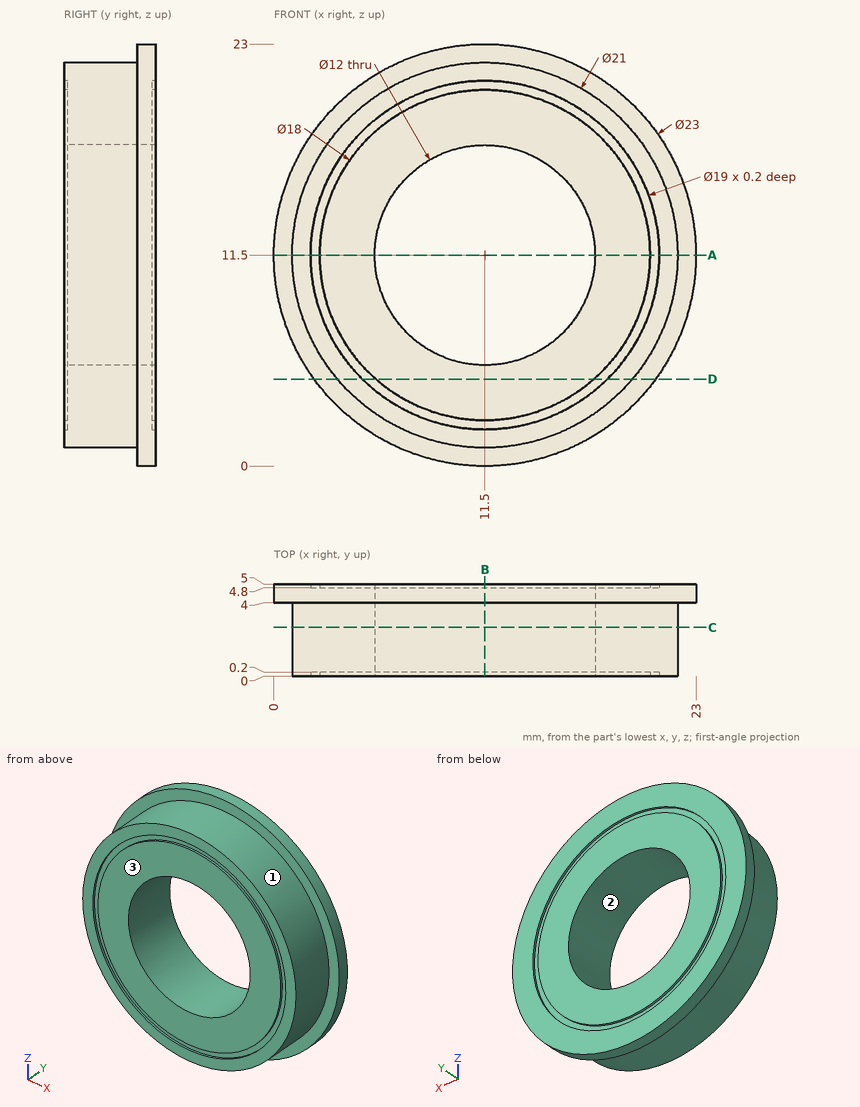
Drawing for the job (mm, zero at the part's lowest x, y, z). Coordinates: 2 decimals unless noted, no trailing zeros. Write each loop counter-clockwise with the first axis right and the second up, starting at its lowest first coordinate (ties: lowest second). Pieces come first, ordered by that corner, then holes. Notation, with made-up numbers: (-8.75, 2.25) -> (11.25, 2.25) arc R23 cw to (11.25, 19.25) -> close; hole circle Ø11 at (54.25, 30.25). An arc over 180 degrees is marked (long way). One line per item, written item: value. Start each with the question number.
1) Slice it at C-C on y = 2.65. Write the cut outline in (x, z).
2) Pull direction X, two halves, no side cores. Call the marked faces 1, 2 and 3: +X half, -X half, draft (parallel to the pull), parting line (faces both ways), or undercut.
3) Flat gauge pins, fed straight in: pin 1 Ø1 at (x, y) = (15.5, 1.5) entering from -Z; pin 2 Ø1.5 at (x, y) = (5, 1) entering from +Z. Where does each tip first touch, or does it go through?
4) Slice it at B-B on x = 11.5. Write the cut outline in (y, z), then the cut area to 3 significant figures.
5) Probe probe 1 along X at (y, z) = (4.9, 11.5); probe 2 along X at (y, z) = (0.15, 11.5); probe 3 along X at (y, z) = (2.5, 11.5). List the from-to ranges inside material, lowest first.
6) Slice it at D-D on z = 4.75. Write the cut outline in (x, y).
7) Slice it at A-A on z = 11.5. Write the cut outline in (x, y), then the cut area to 3 significant figures.
Answers follow:
1. outline: circle Ø21 at (11.5, 11.5); hole circle Ø12 at (11.5, 11.5)
2. face 1: parting line
2. face 2: undercut
2. face 3: draft
3. pin 1: z = 1.6
3. pin 2: z = 20.29
4. outline: (0, 1) -> (4, 1) -> (4, 0) -> (5, 0) -> (5, 2) -> (4.8, 2) -> (4.8, 2.5) -> (5, 2.5) -> (5, 5.5) -> (0, 5.5) -> (0, 2.5) -> (0.2, 2.5) -> (0.2, 2) -> (0, 2) -> close; (0, 17.5) -> (5, 17.5) -> (5, 20.5) -> (4.8, 20.5) -> (4.8, 21) -> (5, 21) -> (5, 23) -> (4, 23) -> (4, 22) -> (0, 22) -> (0, 21) -> (0.2, 21) -> (0.2, 20.5) -> (0, 20.5) -> close
4. area: 46.6 mm2
5. probe 1: 0 to 2, 2.5 to 5.5, 17.5 to 20.5, 21 to 23
5. probe 2: 1 to 2, 2.5 to 5.5, 17.5 to 20.5, 21 to 22
5. probe 3: 1 to 5.5, 17.5 to 22
6. outline: (2.19, 4) -> (3.46, 4) -> (3.46, 0) -> (4.82, 0) -> (4.82, 0.2) -> (5.55, 0.2) -> (5.55, 0) -> (17.45, 0) -> (17.45, 0.2) -> (18.18, 0.2) -> (18.18, 0) -> (19.54, 0) -> (19.54, 4) -> (20.81, 4) -> (20.81, 5) -> (18.18, 5) -> (18.18, 4.8) -> (17.45, 4.8) -> (17.45, 5) -> (5.55, 5) -> (5.55, 4.8) -> (4.82, 4.8) -> (4.82, 5) -> (2.19, 5) -> close
7. outline: (0, 4) -> (1, 4) -> (1, 0) -> (2, 0) -> (2, 0.2) -> (2.5, 0.2) -> (2.5, 0) -> (5.5, 0) -> (5.5, 5) -> (2.5, 5) -> (2.5, 4.8) -> (2, 4.8) -> (2, 5) -> (0, 5) -> close; (17.5, 0) -> (20.5, 0) -> (20.5, 0.2) -> (21, 0.2) -> (21, 0) -> (22, 0) -> (22, 4) -> (23, 4) -> (23, 5) -> (21, 5) -> (21, 4.8) -> (20.5, 4.8) -> (20.5, 5) -> (17.5, 5) -> close
7. area: 46.6 mm2
